Verification items for the finished model (mm, model axes). A direction names the side the tool comes from. Coordinates: 2 decimals unless noted, no trailing zeros. Write each loop counter-clockwise with the first axis right and the second up, starting at its lowest first coordinate (ties: lowest second). Pieces come first, ordered by that corner, then holes. Notation, with made-up numbers: (-9.75, 54.25) -> (-0.75, 54.25) arc R29 ccw to (-0.75, 93.25) -> close; hole circle Ø10 at (52.25, 23). An arc over 180 degrees is marked (long way). Write each question's results on one line, items separated by ' | '. Start each with the question number.
from build123d import *

# Parameters (mm, degrees)
BATON_DEPTH       = 2.54
SKETCH2_R         = 1.27
JOIN_DEPTH        = 6.35
SKETCH4_R         = 2.54
JOINER_CAP_DEPTH  = 2.54
SKETCH5_R         = 1.905
JOINER_HOLE_DEPTH = 2.54


with BuildPart() as part:
    # Sketch1 → baton (new body)
    with BuildSketch(Plane(origin=(0, 0, 0), x_dir=(1, 0, 0), z_dir=(0, 1, 0))):
        with BuildLine():
            Line((-12.7, 5.08), (12.7, 5.08))
            ThreePointArc((12.7, 5.08), (17.78, 0), (12.7, -5.08))
            Line((12.7, -5.08), (-12.7, -5.08))
            ThreePointArc((-12.7, -5.08), (-17.78, 0), (-12.7, 5.08))
        make_face()
    extrude(amount=BATON_DEPTH)

    # Sketch2 → join (add)
    with BuildSketch(Plane(origin=(0, 2.54, 0), x_dir=(1, 0, 0), z_dir=(0, 1, 0))):
        with Locations(Location((-13.97, 0, 0), (0, 0, 270))):
            Circle(SKETCH2_R)
    extrude(amount=JOIN_DEPTH)

    # Sketch4 → joiner cap (add)
    with BuildSketch(Plane(origin=(0, 8.89, 0), x_dir=(1, 0, 0), z_dir=(0, 1, 0))):
        with Locations(Location((-13.97, 0, 0), (0, 0, 270))):
            Circle(SKETCH4_R)
    extrude(amount=JOINER_CAP_DEPTH)

    # Sketch5 → joiner hole (cut)
    with BuildSketch(Plane(origin=(0, 2.54, 0), x_dir=(1, 0, 0), z_dir=(0, 1, 0))):
        with Locations(Location((13.97, 0, 0), (0, 0, 270))):
            Circle(SKETCH5_R)
    extrude(amount=-JOINER_HOLE_DEPTH, mode=Mode.SUBTRACT)


solid = part.part
1. Tool access check on faces 4 (the cylindrical face through (17.78, 1.25, -0.11)), 5 (the cylindrical face through (-16.45, 10.14, -0.55)), 6 (the flat face through (-15, 8.89, 1)). Record the directions out of +Z, -Z, +X, -X, +Y, -Y that give a thin tool (end or side, any length) a straight path to the whole face; none if there is none.
2. Sectioned sample at A-A on z = 0. Record the cut outline in (x, y) (3 decimals).
3. Sectioned sample at B-B on y = 2. Record the cut outline in (x, z) (3 decimals), plus the area to 3 significant figures.
4. Sectioned sample at D-D on x = 6.5. Record the cut outline in (y, z).
5. Mould release check, pull along Y, two halves, no side actions. Record for faces 1 (the flat face through (0, 1, -5.08)), 2 (the cylindrical face through (-12.71, 5.67, -0.17)), 3 (the flat face through (-14, 11.43, 0)): +Y half, -Y half, draft (parallel to the pull), parting line (faces both ways), or undercut.
6. Depth check by flat-ended pin: pin 1 Ø2 at (y, z) = (6, -0.5) entering from -X; pin 2 Ø1 at (y, z) = (9.5, 1) entering from +X; pin 3 Ø6 at (y, z) = (3, -4) entering from +X. Enter the tip coordinate at first touch or a pass-through.
7. Sectioned sample at C-C on x = 13.97. Record the cut outline in (y, z) (3 decimals).
8. Material ranges on probe 1 along X at (y, z) = (1.75, 0) (3 decimals); probe 2 along Y at (x, z) = (2, 1.75); probe 3 along X at (y, z) = (5.5, -0.5), recorded low to high. Write a range as from..to.
Computed values:
1) face 4: +X, +Y, -Y | face 5: +Y | face 6: none
2) outline: (-17.78, 0) -> (12.065, 0) -> (12.065, 2.54) -> (-12.7, 2.54) -> (-12.7, 8.89) -> (-11.43, 8.89) -> (-11.43, 11.43) -> (-16.51, 11.43) -> (-16.51, 8.89) -> (-15.24, 8.89) -> (-15.24, 2.54) -> (-17.78, 2.54) -> close; (15.875, 0) -> (17.78, 0) -> (17.78, 2.54) -> (15.875, 2.54) -> close
3) outline: (-12.7, -5.08) -> (12.7, -5.08) arc R5.08 ccw to (12.7, 5.08) -> (-12.7, 5.08) arc R5.08 ccw to start; hole circle Ø3.81 at (13.97, 0) | area: 328 mm^2
4) outline: (0, -5.08) -> (2.54, -5.08) -> (2.54, 5.08) -> (0, 5.08) -> close
5) face 1: draft | face 2: undercut | face 3: +Y half
6) pin 1: stops at x = -15.24 | pin 2: stops at x = -11.48 | pin 3: stops at x = 17.67
7) outline: (0, -4.919) -> (2.54, -4.919) -> (2.54, -1.905) -> (0, -1.905) -> close; (0, 1.905) -> (2.54, 1.905) -> (2.54, 4.919) -> (0, 4.919) -> close
8) probe 1: x = -17.78..12.065, 15.875..17.78 | probe 2: y = 0..2.54 | probe 3: x = -15.14..-12.8
